Check sheet for the modelled part. Datum: model origin and axes. Units: mm. Coordinates: 2 decimals unless noted, no trailing zeros. Loops run counter-clockwise (first coordinate to the right, second up) from the corner with the lowest first, then second, coordinate; pieces in that order, holes last. Notation, with made-up numbers: (29, -5.5) -> (60, -5.5) arc R19 cw to (60, 14.5) -> close; hole circle Ø5 at (74.5, 50.5). An arc over 180 degrees is marked (long way). Use CSV: the item, a comma, the result in double quotes. Start each with the question number.
1. Thickness scan on L1, parallel to X at y = -34.5, z = -1.95 (3 decimals); L2, parallel to Y at x = -80.5, z = -0.85. Record the ranges inside material, lowest first.
2. Gauge pin test, flat ends, axial feed: pin 1 (1.5 mm diameter, centred on x = -28, y = 19.5, fed in from +Z); pin 2 (1 mm diameter, centred on x = 108, z = -1.5, fed in from +Y); pin 3 (1 mm diameter, centred on x = -108.5, z = -2, fed in from -Y); pin 4 (2.5 mm diameter, centred on x = -100.59, y = 7, fed in from +Z). Record the tip position at first contact, or that the pin passes through.
3. Sectioned sample at B-B, the plane x = -73.5. Record the cut outline in (y, z) (3 decimals).
4. Sectioned sample at A-A, the plane z = -2.05. Count the separate pieces of the cut face and the enclosed holes in it, and give its area (3 significant figures).
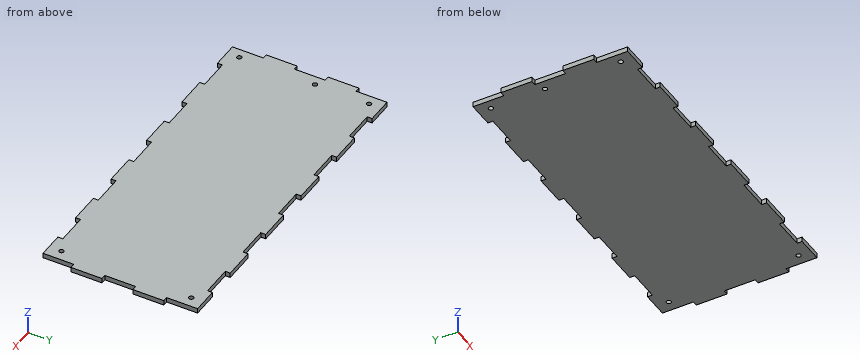
```python
from build123d import *

# Parameters (mm, degrees)
SKETCH51_W           = 220
SKETCH51_H           = 99.999981374
SKETCH51_R           = 1.5
BOSS_EXTRUDE13_DEPTH = 3.175
SKETCH52_W           = 3.175
SKETCH52_H           = 20
SKETCH52_W_2         = 20
SKETCH52_H_2         = 3.175
CUT_EXTRUDE25_DEPTH  = 3.175


with BuildPart() as part:
    # Sketch51 → Boss-Extrude13 (new body)
    with BuildSketch(Plane(origin=(0, 0, 0), x_dir=(-1, 0, 0), z_dir=(0, 0, -1))):
        with Locations((4.414e-06, 4.4643e-05)):
            Rectangle(SKETCH51_W, SKETCH51_H)
        with Locations((100.587627215, -41.999946044)):
            Circle(SKETCH51_R, mode=Mode.SUBTRACT)
        with Locations((100.587627215, 42.00003533)):
            Circle(SKETCH51_R, mode=Mode.SUBTRACT)
        with Locations((-99.9999958, -41.999946044)):
            Circle(SKETCH51_R, mode=Mode.SUBTRACT)
        with Locations((-99.9999958, 42.00003533)):
            Circle(SKETCH51_R, mode=Mode.SUBTRACT)
        with Locations((100.587627215, 7.000053956)):
            Circle(SKETCH51_R, mode=Mode.SUBTRACT)
    extrude(amount=BOSS_EXTRUDE13_DEPTH)

    # Sketch52 → Cut-Extrude25 (cut)
    with BuildSketch(Plane(origin=(0, 0, -3.175), x_dir=(-1, 0, 0), z_dir=(0, 0, -1))):
        with Locations((108.4125042, 3.533e-05)):
            Rectangle(SKETCH52_W, SKETCH52_H)
        with Locations((108.4125042, 40.00003533)):
            Rectangle(SKETCH52_W, SKETCH52_H)
        with Locations((108.4125042, -39.99996467)):
            Rectangle(SKETCH52_W, SKETCH52_H)
        with Locations((-108.4124958, 3.533e-05)):
            Rectangle(SKETCH52_W, SKETCH52_H)
        with Locations((-108.4124958, 40.00003533)):
            Rectangle(SKETCH52_W, SKETCH52_H)
        with Locations((-108.4124958, -39.99996467)):
            Rectangle(SKETCH52_W, SKETCH52_H)
        with Locations((40.0000042, 48.41253533)):
            Rectangle(SKETCH52_W_2, SKETCH52_H_2)
        with Locations((80.0000042, 48.41253533)):
            Rectangle(SKETCH52_W_2, SKETCH52_H_2)
        with Locations((4.2e-06, 48.41253533)):
            Rectangle(SKETCH52_W_2, SKETCH52_H_2)
        with Locations((-39.9999958, 48.41253533)):
            Rectangle(SKETCH52_W_2, SKETCH52_H_2)
        with Locations((-79.9999958, 48.41253533)):
            Rectangle(SKETCH52_W_2, SKETCH52_H_2)
        with Locations((40.0000042, -48.412446044)):
            Rectangle(SKETCH52_W_2, SKETCH52_H_2)
        with Locations((80.0000042, -48.412446044)):
            Rectangle(SKETCH52_W_2, SKETCH52_H_2)
        with Locations((4.2e-06, -48.412446044)):
            Rectangle(SKETCH52_W_2, SKETCH52_H_2)
        with Locations((-39.9999958, -48.412446044)):
            Rectangle(SKETCH52_W_2, SKETCH52_H_2)
        with Locations((-79.9999958, -48.412446044)):
            Rectangle(SKETCH52_W_2, SKETCH52_H_2)
    extrude(amount=-CUT_EXTRUDE25_DEPTH, mode=Mode.SUBTRACT)


solid = part.part
```
Completed:
1,L1,"-106.825 to 106.825"
1,L2,"-46.82 to 46.83"
2,pin 1,"z = 0"
2,pin 2,"y = 30"
2,pin 3,"y = -30"
2,pin 4,"through"
3,outline,"(-46.825, -3.175) -> (46.825, -3.175) -> (46.825, 0) -> (-46.825, 0) -> close"
4,separate pieces,"1"
4,enclosed holes,"5"
4,area,"20,900 mm²"
